from build123d import *

# Parameters (mm, degrees)
F0_R     = 6
F0_R_2   = 4.075
F1_DEPTH = 3
F2_SIZE  = 0.2
F3_SIZE2 = 0.267949
F3_SIZE  = 1


with BuildPart() as f1:
    # F0 (on Top) → F1 (new body)
    with BuildSketch(Plane.XY):
        Circle(F0_R)
        Circle(F0_R_2, mode=Mode.SUBTRACT)
    extrude(amount=F1_DEPTH)

    # F2
    f2_edges = [f1.edges().sort_by_distance(p)[0] for p in [
        (-4.075, 0, 3),
        (-6, 0, 0),
        (-6, 0, 3),
    ]]
    chamfer(f2_edges, length=F2_SIZE)

    # F3
    f3_edges = [f1.edges().sort_by_distance(p)[0] for p in [
        (-4.075, 0, 0),
    ]]
    chamfer(f3_edges, length=F3_SIZE, length2=F3_SIZE2)


solid = f1.part
Geometry check sheet. Reference: the model listing, model coordinates, mm. Give positions to 0.01 mm unless a question says otherwise; leave off trailing zeros. Write each loop counter-clockwise with the first axis right and the second up, starting at its lowest first coordinate (ties: lowest second). Pieces come first, ordered by that corner, then holes. Notation, with made-up numbers: M -30.75,-1 L -18.75,-1 A23 cw -18.75,35 Z; hole C 6,-27 d1. An arc over 180 degrees is marked long. One line per question, with ' | ' between items.
1. Mould release check, pull along Y, two halves, no side actions. Record for faces 1 (the face through (-3.234, -2.48, 1.516)), 2 (the face through (-2, -4, 3)), 3 (the face through (-6, 0, 1)): released by +Y, released by -Y, zero draft, split by the parting line, or undercut.
Ans:
face 1: undercut | face 2: zero draft | face 3: split by the parting line
2. Cross-section at A-A (y = 0). Enter the section's corners in (x, z) (3 decimals).
Ans:
outline: M -6,0.2 L -5.8,0 L -5.075,0 L -4.075,0.268 L -4.075,2.8 L -4.275,3 L -5.8,3 L -6,2.8 Z; M 4.075,0.268 L 5.075,0 L 5.8,0 L 6,0.2 L 6,2.8 L 5.8,3 L 4.275,3 L 4.075,2.8 Z
3. Gauge pin test, flat ends, axial feed: pin 1 (1 mm diameter, centred on y = -2.5, z = 2, fed in from -X); pin 2 (5 mm diameter, centred on x = 3.5, y = 1, fed in from -Z). Record the tip position at first contact, or that the pin passes through.
Ans:
pin 1: x = -5.66 | pin 2: z = 0
4. Scan lines: line 1 along Y through (x, z) = (0, 1.3) (3 decimals); line 2 along X through (y, z) = (-0.5, 0.7). Record each from-to range of solid material in increasing order. Write a range as from..to.
Ans:
line 1: -6..-4.075, 4.075..6 | line 2: -5.98..-4.04, 4.04..5.98
5. Cross-section at C-C (z = 1). Enter the section's corners in (x, y) (3 decimals).
Ans:
outline: C 0,0 d12; hole C 0,0 d8.15
